CAD build for the part. Positions are in the model's coordinates, mm. Face numbers are marked on the shaded views. A direction names the side the tool comes from. Give positions to 0.01 mm unless a question says otherwise; leave off trailing zeros. Loops run counter-clockwise (first coordinate to the right, second up) from the corner with the lowest first, then second, coordinate; pieces in that order, holes last. Notation, with made-up numbers: M 78.25,81 L 132.25,81 A23 cw 132.25,113 Z; hole C 86,29.5 d11. An arc over 180 degrees is marked long. Answer as CSV lines item,"result".
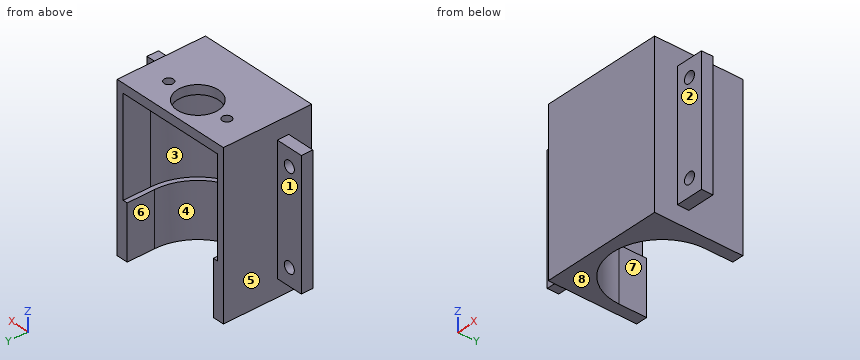
Autodesk Inventor part; units mm, degrees
ref_plane "작업 평면1" through (0, 10, 4) normal (0, -1, 0) x (1, 0, 0)
ref_plane "YZ Plane" through (0, 0, 0) normal (1, 0, 0) x (0, 1, 0)
ref_plane "XZ Plane" through (0, 0, 0) normal (0, 1, 0) x (-1, 0, 0)
sketch "스케치1" plane through (0, 0, 0) normal (0, 0, 1) x (1, 0, 0)
  line L0 (0, 0) -> (53, 0)
  line L1 (53, 0) -> (53, 38.5)
  line L2 (53, 38.5) -> (0, 38.5)
  line L3 (0, 38.5) -> (0, 0)
  arc A0 (3, 26.5) -> (6.2948, 38.5) centre (26.5, 26.5) ccw
  circle A1 centre (12, 26.5) radius 2
  circle A2 centre (41, 26.5) radius 2
  arc A3 (5, 26.5) -> (8.6604, 38.5) centre (26.5, 26.5) ccw
  circle A4 centre (26.5, 26.5) radius 9
  line L4 (3, 38.5) -> (3, 26.5)
  line L5 (5, 38.5) -> (5, 26.5)
  line L6 (48, 51.0228) -> (48, 26.5)
  line L7 (50, 50.0136) -> (50, 26.5)
  line L8 (26.5, 0) -> (26.5, 1.4842)
  line L9 (0, 28) -> (-15, 28)
  line L10 (-15, 28) -> (-15, 13)
  line L11 (-15, 13) -> (0, 13)
  circle A5 centre (-9, 20.5) radius 2.5
  line L12 (53, 28) -> (68, 28)
  line L13 (68, 28) -> (68, 13)
  line L14 (68, 13) -> (53, 13)
  circle A6 centre (62, 20.5) radius 2.5
  circle A7 centre (-9, 20.5) radius 5
  circle A8 centre (62, 20.5) radius 5
  point P0 (44.3396, 38.5)
  point P1 (8.6604, 38.5)
  point P2 (6.2948, 38.5)
  point P3 (46.7052, 38.5)
  point P4 (50, 38.5)
  point P5 (48, 38.5)
  point P6 (-15, 20.5)
  dimension "d1" = 47
  dimension "d2" = 3
  dimension "d3" = 3
  dimension "d4" = 3
  dimension "d5" = 4
  dimension "d6" = 29
  dimension "d7" = 14.5
  dimension "d8" = 10
  dimension "d9" = 43
  dimension "d16" = 18
  dimension "d23" = 15
  dimension "d24" = 15
  dimension "d25" = 6
  dimension "d26" = 5
  dimension "d27" = 13
  dimension "d30" = 10
extrude "돌출1" add sketch "스케치1" along normal blind 4 contours L3 L2 L4 A0 L7 L1 L0 | L2 L5 A3 L6 A0 L4 | L2 A3 L5 | L7 A0 L6 L2 | L6 A0 L2 | A0 L6 A3 L2
extrude "돌출2" add sketch "스케치1" against normal blind 66 contours L3 L2 L4 A0 L7 L1 L0 | L2 L5 A3 L6 A0 L4 | L7 A0 L6 L2
extrude "돌출3" cut sketch "스케치1" against normal blind 42.5 contours L2 L5 A3 L6 A0 L4 | L2 A3 L5 | L7 A0 L6 L2 | L6 A0 L2 | A0 L6 A3 L2 | A1 | A2 | A4
ref_plane "작업 평면1" through (0, 10, 4) normal (0, -1, 0) x (1, 0, 0)
sketch "스케치2" plane through (0, 10, 4) normal (0, -1, 0) x (1, 0, 0)
  line L0 (0, -70) -> (0, 0)
  line L1 (0, 0) -> (0, -70)
  line L2 (0, 0) -> (53, 0)
  line L3 (53, 0) -> (0, 0)
  line L4 (10, 0) -> (14, 0)
  line L5 (39, 0) -> (43, 0)
  line L6 (17.5, 0) -> (35.5, 0)
  line L7 (53, -70) -> (53, 0)
  line L8 (53, -70) -> (53, 0)
  line L9 (0, -7.5) -> (-12, -7.5)
  line L10 (-12, -7.5) -> (-12, -62.5)
  line L11 (-12, -62.5) -> (0, -62.5)
  circle A0 centre (-6, -15) radius 2.5
  circle A1 centre (-6, -55) radius 2.5
  line L12 (26.5, 0) -> (26.5, -15)
  line L13 (53, -7.5) -> (65, -7.5)
  line L14 (65, -7.5) -> (65, -62.5)
  line L15 (65, -62.5) -> (53, -62.5)
  circle A2 centre (59, -15) radius 2.5
  circle A3 centre (59, -55) radius 2.5
  point P0 (0, -4)
  point P1 (-6, -62.5)
  point P2 (0, -35)
  point P3 (-12, -35)
  dimension "d36" = 5
  dimension "d37" = 5
  dimension "d39" = 55
  dimension "d40" = 12
  dimension "d41" = 40
  dimension "d42" = 20
extrude "돌출6" add sketch "스케치2" against normal blind 5
equation "\"d7\" = 0.5 * d6"
properties part number "MotorCover_3D 인쇄"
Q1. Cut at A-A (z = -11). Write the cut outline in (x, y).
Solution:
outline,"M -12,10 L -8.5,10 L -8.5,15 L -12,15 Z; M -3.5,10 L 0,10 L 0,0 L 53,0 L 53,10 L 56.5,10 L 56.5,15 L 53,15 L 53,38.5 L 50,38.5 L 50,26.5 A23.5 cw 3,26.5 L 3,38.5 L 0,38.5 L 0,15 L -3.5,15 Z; M 61.5,10 L 65,10 L 65,15 L 61.5,15 Z"
Q2. Cut at D-D (x = -6). Write the cut outline in (y, z).
Solution:
outline,"M 10,-58.5 L 15,-58.5 L 15,-53.5 L 10,-53.5 Z; M 10,-48.5 L 15,-48.5 L 15,-13.5 L 10,-13.5 Z; M 10,-8.5 L 15,-8.5 L 15,-3.5 L 10,-3.5 Z"
Q3. Wall check: line 1 (Z direction, x = -6, y = 12); line 2 (X direction, y = 27, z = -24); line 3 (Z direction, x = 49, y = 32.5). Give the ranges that are in metal, low to high. Write a range as [from, to].
Solution:
line 1,"z = [-58.5, -53.5], [-48.5, -13.5], [-8.5, -3.5]"
line 2,"x = [0, 3], [50, 53]"
line 3,"z = [-66, -42.5], [0, 4]"
Q4. Which spindle directions (+Z, -Z, +X, -X, +Y, -Y) get a long thin tool onto all of the face, cutting with end or side? Do the marked faces 1, 2, 3 and 4. Say none if no direction does.
Solution:
face 1,"+Z, -Z, -X, +Y"
face 2,"+Z, -Z, +X, -Y"
face 3,"+Y"
face 4,"-Z, +Y"
Q5. Pin check, flat tips, straight feed: P1, Ø4, axis at x = -7.5, y = 11.5, coming from the -Z side; P2, Ø6, axis at x = 58.5, z = -21, coming from the -Y side; P3, Ø4, axis at x = 60, y = 11.5, coming from the +Z side; P4, Ø6, axis at x = 1, z = -36, coming from the -Y side. Stop position of each tip, or through.
Solution:
P1,"stops at z = -58.5"
P2,"stops at y = 10"
P3,"stops at z = -3.5"
P4,"stops at y = 0"
Q6. Cut at B-B (x = 26.5). Write the cut outline in (y, z).
Solution:
outline,"M 0,-66 L 5,-66 L 5,-42.5 L 3,-42.5 L 3,0 L 17.5,0 L 17.5,4 L 0,4 Z; M 35.5,0 L 38.5,0 L 38.5,4 L 35.5,4 Z"
Q7. Cut at C-C (y = 32.5). Write the cut outline in (x, z), and give its area (3 significant figures).
Solution:
outline,"M 0,-66 L 5,-66 L 5,-42.5 L 3,-42.5 L 3,0 L 19.79,0 L 19.79,4 L 0,4 Z; M 33.21,0 L 50,0 L 50,-42.5 L 48,-42.5 L 48,-66 L 53,-66 L 53,4 L 33.21,4 Z"
area,"648 mm²"
Q8. Mould opens along X. For the marked faces 5, 6, 7 and 8 say: released by +X, released by -X, zero draft, split by the parting line, or undercut.
Solution:
face 5,"released by -X"
face 6,"undercut"
face 7,"undercut"
face 8,"zero draft"
